```python
from build123d import *

# Parameters (mm, degrees)
SKETCH_1_W          = 22
SKETCH_1_H          = 22
SKETCH_1_R          = 1.55
EXTRUDE_1_DEPTH     = 5
EXTRUDE_2_DEPTH     = 127
SKETCH_3_W          = 4
SKETCH_3_H          = 8
EXTRUDE_3_DEPTH     = 34
EXTRUDE_4_DEPTH     = 5
SKETCH_7_W          = 3.1
SKETCH_7_H          = 40
CUT_EXTRUDE_3_DEPTH = 5


with BuildPart() as part:
    # 草图1 → 凸台-拉伸1 (new body)
    with BuildSketch(Plane(origin=(0, 0, 0), x_dir=(1, 0, 0), z_dir=(0, 1, 0))):
        Rectangle(SKETCH_1_W, SKETCH_1_H)
        with Locations(Location((-7.424621202, 7.424621202, 0), (0, 0, 270))):
            Circle(SKETCH_1_R, mode=Mode.SUBTRACT)
        with Locations(Location((7.424621202, 7.424621202, 0), (0, 0, 270))):
            Circle(SKETCH_1_R, mode=Mode.SUBTRACT)
        with Locations(Location((7.424621202, -7.424621202, 0), (0, 0, 270))):
            Circle(SKETCH_1_R, mode=Mode.SUBTRACT)
        with Locations(Location((-7.424621202, -7.424621202, 0), (0, 0, 270))):
            Circle(SKETCH_1_R, mode=Mode.SUBTRACT)
    extrude(amount=EXTRUDE_1_DEPTH)

    # 草图2 → 凸台-拉伸2 (add)
    with BuildSketch(Plane(origin=(0, 5, 0), x_dir=(1, 0, 0), z_dir=(0, 1, 0))):
        Polygon((0, 6), (-6, 0), (0, -6), (6, 0), align=None)
    extrude(amount=EXTRUDE_2_DEPTH)

    # 草图3 → 凸台-拉伸3 (add)
    with BuildSketch(Plane(origin=(-3, 0, 3), x_dir=(0.7071067811865452, 0, 0.7071067811865498), z_dir=(-0.7071067811865498, 0, 0.7071067811865452))):
        with Locations((0, 64)):
            Rectangle(SKETCH_3_W, SKETCH_3_H)
    extrude(amount=EXTRUDE_3_DEPTH)

    # 草图4 → 凸台-拉伸4 (add)
    with BuildSketch(Plane(origin=(-3, 0, 3), x_dir=(0.7071067811865452, 0, 0.7071067811865498), z_dir=(-0.7071067811865498, 0, 0.7071067811865452))):
        Polygon((4.242640687, 132), (25, 132), (25, 90), (-25, 90), (-25, 132), align=None)
    extrude(amount=EXTRUDE_4_DEPTH)

    # 草图7 → 切除-拉伸3 (cut)
    with BuildSketch(Plane(origin=(-6.535533906, 0, 6.535533906), x_dir=(0.7071067811865454, 0, 0.7071067811865498), z_dir=(-0.7071067811865498, 0, 0.7071067811865454))):
        with Locations((-14.73, 111)):
            Rectangle(SKETCH_7_W, SKETCH_7_H)
        with Locations((14.73, 111)):
            Rectangle(SKETCH_7_W, SKETCH_7_H)
    extrude(amount=-CUT_EXTRUDE_3_DEPTH, mode=Mode.SUBTRACT)


solid = part.part
```
Build history of the part. All positions in model axes, mm. A direction names the side the tool comes from. Round coordinates to 2 decimals unless told otherwise and drop trailing zeros. Write each loop counter-clockwise with the first axis right and the second up, starting at its lowest first coordinate (ties: lowest second). Pieces come first, ordered by that corner, then holes.
1) Band-saw the part on C-C, the plane z = 19.5. List the corners of the cut face in (x, y), and give its area (3 significant figures).
2) Band-saw the part on D-D, the plane y = 13.5. List the corners of the cut face in (x, z), and give its area (3 significant figures).
3) Mould opens along X. For faces 1 (the cylindrical face through (7.493, 2.465, 5.876)), 2 (the flat face through (-16.27, 63.94, 13.44)), 3 (the flat face through (0, 2, -11)) say: +X half, -X half, draft (parallel to the pull), parting line (faces both ways), or undercut.
4) Band-saw the part on A-A, the plane y = 122. List the corners of the cut face in (x, z).
5) 3-axis set-ups, long thin cutter, end or side, ignore diameter. For faces 4 (the flat face through (3, 68, 3)), 5 (the cylindrical face through (-6.38, 2.46, 6.28)), 6 (the flat face through (-16.304, 110.72, -6.719)): which of +Z, -Z, +X, -X, +Y, -Y reach the whole face in a straight line?
6) Band-saw the part on B-B, the plane x = -22. List the corners of the cut face in (y, z), and give its area (3 significant figures).
7) Pin check, flat tips, straight feed: pin 1 (5.5 mm diameter, centred on y = 2, z = 3, fed in from +X); pin 2 (8 mm diameter, centred on x = -16.5, y = 57, fed in from +Z); pin 3 (4 mm diameter, centred on y = 67, z = 4.5, fed in from +X); pin 4 (3 mm diameter, centred on x = -7.42, z = -7.42, fed in from -Y). Stop position of each tip, or through.
8) Drill centre lines: probe 1 along Y at (x, z) = (-14.5, 15); probe 2 along Z at (x, y) = (4, 120); probe 3 along Y at (x, z) = (-16, -9). Where is each one in solid material? Low to high.
Ans:
1. outline: (-22.33, 60) - (-16.67, 60) - (-16.67, 68) - (-22.33, 68) - close; (6.43, 90) - (13.5, 90) - (13.5, 132) - (6.43, 132) - close
1. area: 342 mm2
2. outline: (-6, 0) - (0, -6) - (6, 0) - (0, 6) - close
2. area: 72.0 mm2
3. face 1: undercut
3. face 2: -X half
3. face 3: draft
4. outline: (-24.21, -11.14) - (-20.68, -14.68) - (-14.51, -8.51) - (-18.05, -4.98) - close; (-15.86, -2.78) - (-12.32, -6.32) - (-6, 0) - (0, -6) - (6, 0) - (0, 6) - (6.32, 12.32) - (2.78, 15.86) - close; (4.98, 18.05) - (8.51, 14.51) - (14.68, 20.68) - (11.14, 24.21) - close
5. face 4: +X, +Y
5. face 5: -Y
5. face 6: none
6. outline: (60, 19.17) - (68, 19.17) - (68, 24.83) - (60, 24.83) - close; (90, -13.36) - (132, -13.36) - (132, -8.93) - (90, -8.93) - close
6. area: 231 mm2
7. pin 1: stops at x = 11
7. pin 2: stops at z = 21.97
7. pin 3: stops at x = 3.5
7. pin 4: passes through
8. probe 1: y = 60 to 68
8. probe 2: z = -2 to 2, 10 to 14.64
8. probe 3: y = 90 to 132
